Could you check a few things on this model? Use its own coordinates, in mm. Face numbers are marked on the shaded views. A direction names the side the tool comes from. Coordinates: 2 decimals unless noted, no trailing zeros. Write each loop counter-clockwise with the first axis right and the second up, starting at its lowest first coordinate (ties: lowest second). Pieces come first, ordered by that corner, then holes.
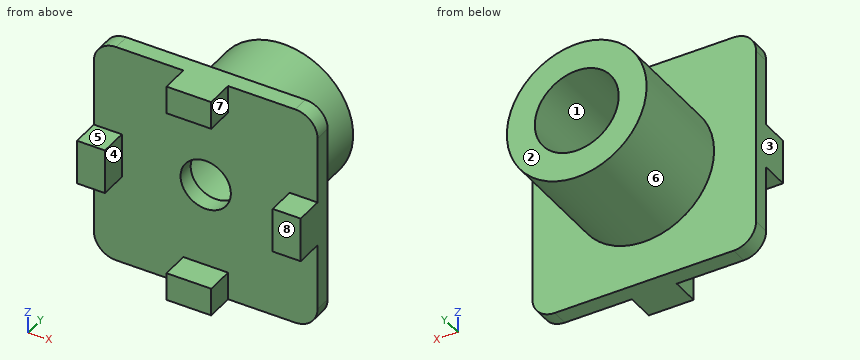
Autodesk Fusion 360 part; units mm, degrees
sketch "Sketch1" plane through (0, 0, 0) normal (0, 1, 0) x (1, 0, 0)
  line L0 (20, -20) -> (-20, -20)
  line L1 (-20, -20) -> (-20, 20)
  line L2 (-20, 20) -> (20, 20)
  line L3 (20, 20) -> (20, -20)
  line L4 (20, -20) -> (-20, 20) construction
  line L5 (-20, -20) -> (20, 20) construction
  line L6 (-20, 4) -> (-15, 4)
  line L7 (-15, 4) -> (-15, -4)
  line L8 (-15, -4) -> (-20, -4)
  line L9 (-20, -4) -> (-20, 4)
  line L10 (-4, 20) -> (4, 20)
  line L11 (4, 20) -> (4, 15)
  line L12 (4, 15) -> (-4, 15)
  line L13 (-4, 15) -> (-4, 20)
  line L14 (20, 4) -> (15, 4)
  line L15 (15, 4) -> (15, -4)
  line L16 (15, -4) -> (20, -4)
  line L17 (20, -4) -> (20, 4)
  line L18 (-4, -20) -> (4, -20)
  line L19 (4, -20) -> (4, -15)
  line L20 (4, -15) -> (-4, -15)
  line L21 (-4, -15) -> (-4, -20)
  dimension "d1" = 40
  dimension "d2" = 40
  dimension "d3" = 5
  dimension "d4" = 8
  dimension "d5" = 16
  dimension "d6" = 5
  dimension "d7" = 16
  dimension "d8" = 8
  dimension "d9" = 5
  dimension "d10" = 5
  dimension "d11" = 8
  dimension "d12" = 8
  dimension "d13" = 16
  dimension "d14" = 16
extrude "Extrude1" add sketch "Sketch1" against normal blind 3 contours L0 L1 L2 L3 L6 L7 L8 L11 L12 L13 L14 L15 L16 L19 L20 L21
extrude "Extrude2" add sketch "Sketch1" against normal blind 8 contours L0 L18 L19 L20 L21 | L3 L14 L15 L16 L17 | L1 L6 L7 L8 L9 | L2 L10 L11 L12 L13
hole "Hole1" at (0, 0, 0) direction (0, -1, 0) diameter 9 depth 30 tip angle 118
fillet "Fillet1" radius 4 4 edges at (20, -1.5, -20) (-20, -1.5, -20) (20, -1.5, 20) (-20, -1.5, 20)
sketch "Sketch2" plane through (0, 0, 0) normal (0, 1, 0) x (-1, 0, 0)
  circle A0 centre (0, 0) radius 4.5
  arc A1 (20, 16) -> (16, 20) centre (16, 16) ccw
  line L0 (16, 20) -> (-16, 20)
  arc A2 (-16, 20) -> (-20, 16) centre (-16, 16) ccw
  line L1 (-20, 16) -> (-20, -16)
  arc A3 (-20, -16) -> (-16, -20) centre (-16, -16) ccw
  line L2 (-16, -20) -> (16, -20)
  arc A4 (16, -20) -> (20, -16) centre (16, -16) ccw
  line L3 (20, -16) -> (20, 16)
  circle A5 centre (0, 0) radius 12.5
  dimension "d24" = 25
extrude "Extrude3" add sketch "Sketch2" along normal blind 20 contours A5
sketch "Sketch3" plane through (0, 20, 0) normal (0, 1, 0) x (-1, 0, 0)
  circle A0 centre (0, 0) radius 4.5
  circle A1 centre (0, 0) radius 12.5
hole "Hole2" at (0, 20, 0) direction (0, -1, 0) diameter 9 depth 40.942 tip angle 118 counterbore diameter 15 counterbore depth 20
equation "d6 = d3"
equation "d7 = d5"
equation "d8 = d4"
equation "d9 = d3"
equation "d10 = d3"
equation "d11 = d4"
equation "d12 = d4"
equation "d13 = d7"
equation "d14 = d7"
1. I want a section at A-A on y = -5. Please give me the cut outline in (x, z), plus the area to 3 significant figures.
Verdict:
outline: (-20, -4) - (-15, -4) - (-15, 4) - (-20, 4) - close; (-4, -20) - (4, -20) - (4, -15) - (-4, -15) - close; (-4, 15) - (4, 15) - (4, 20) - (-4, 20) - close; (15, -4) - (20, -4) - (20, 4) - (15, 4) - close
area: 160 mm2
2. I want a section at B-B on x = 0. Please give me the cut outline in (y, z).
Verdict:
outline: (-8, -20) - (0, -20) - (0, -12.5) - (20, -12.5) - (20, -7.5) - (0, -7.5) - (0, -4.5) - (-3, -4.5) - (-3, -15) - (-8, -15) - close; (-8, 15) - (-3, 15) - (-3, 4.5) - (0, 4.5) - (0, 7.5) - (20, 7.5) - (20, 12.5) - (0, 12.5) - (0, 20) - (-8, 20) - close
3. I want a section at D-D on z = 0. Please give me the cut outline in (x, y), plus the area to 3 significant figures.
Verdict:
outline: (-20, -8) - (-15, -8) - (-15, -3) - (-4.5, -3) - (-4.5, 0) - (-7.5, 0) - (-7.5, 20) - (-12.5, 20) - (-12.5, 0) - (-20, 0) - close; (4.5, -3) - (15, -3) - (15, -8) - (20, -8) - (20, 0) - (12.5, 0) - (12.5, 20) - (7.5, 20) - (7.5, 0) - (4.5, 0) - close
area: 343 mm2
4. If we mould it in two halves opening along X, with no side actions, what happens to the marked faces 1, 2, 3 and 4? For each: pulls with the +X half, pulls with the -X half, needs draft (parallel to the pull), parting line crosses it, or undercut.
Verdict:
face 1: undercut
face 2: needs draft
face 3: pulls with the -X half
face 4: undercut
5. For pin 1 (12 mm diameter, centred on x = 0.5, z = -4.5, fed in from -Y); pin 2 (2.5 mm diameter, centred on y = -4.5, z = -18.5, fed in from +X); pin 3 (3 mm diameter, centred on x = 4.5, y = 3.5, fed in from +Z), each with a flat end and sliding along its axis, tell me the tip position at first contact or that it passes through.
Verdict:
pin 1: stops at y = -3
pin 2: stops at x = 4
pin 3: stops at z = 12.13
6. I want a section at C-C on y = -1.75. Please give me the cut outline in (x, z).
Verdict:
outline: (-20, -16) arc R4 ccw to (-16, -20) - (16, -20) arc R4 ccw to (20, -16) - (20, 16) arc R4 ccw to (16, 20) - (-16, 20) arc R4 ccw to (-20, 16) - close; hole circle Ø9 at (0, 0)
7. On a 3-axis mill with a long thin cutter (end or side, diameter ignored), from which of +Z, -Z, +X, -X, +Y, -Y can I reach the whole of each face in a straight line? I mean the marked faces 5, 6, 7 and 8. Say none if no direction works.
Verdict:
face 5: +Z, +X, -X, -Y
face 6: +Y
face 7: +Z, -Z, +X, -Y
face 8: +Z, -Z, +X, -X, -Y
8. Please list where these lines run through material, in increasing order: line 1 along Z through (x, y) = (0, 8); line 2 along X through (y, z) = (-0.95, 0).
Verdict:
line 1: z = -12.5 to -7.5, 7.5 to 12.5
line 2: x = -20 to -4.5, 4.5 to 20
